Read the model definition and answer for the solid it produces. Units are mm, in the model's axes. A direction names the side the tool comes from. Give positions to 0.01 mm unless a question says otherwise; leave off trailing zeros. Loops run counter-clockwise (first coordinate to the right, second up) from the corner with the lowest first, then second, coordinate; pieces in that order, holes last. Notation, with made-up numbers: (81.5, 13.25) - (87.5, 13.25) arc R5 cw to (87.5, 20.25) - close; hole circle Ø8 at (6.25, -30). An arc over 180 degrees is marked (long way). Use a Markdown table: item, result. Add a question column.
Item 1: A cutting plane is placed at A-A (x = 0). Determine the outline of the cut face in (y, z), plus the area to 3 significant figures.
Item 2: Which of the six approach directions +Z, -Z, +X, -X, +Y, -Y give full straight-line access (tool end or side, diameter ignored) to faces 4 (the face through (19.48, 3.76, -21.04)), 5 (the face through (-26, 32, 12.7)), 6 (the face through (20.863, 59.743, -21.474))?
Item 3: Consider probe 1 along Z at (x, y) = (0, 49); probe 2 along Y at (x, z) = (-23, 12). Determine where each line is inside the solid, lowest interval first. Write a range as [from, to].
Item 4: A cutting plane is placed at C-C (y = 44.5). Determine the outline of the cut face in (x, z).
Item 5: Each of these flat-tipped pins is pushed along its axis until it touches: P1, Ø12, axis at x = -2.5, y = 45, coming from the +Z side; P2, Ø2, axis at x = -20.43, z = 20.43, coming from the +Y side; P3, Ø8, axis at x = -24.5, y = 29.5, coming from the -Z side; P4, Ø13.5, axis at x = 12.5, z = -18, coming from the -Y side. Where does it stop, or does it pass through?
Item 6: A cutting plane is placed at B-B (z = 0). Determine the outline of the cut face in (x, y), plus the area to 3 significant figures.
Item 7: A cutting plane is placed at D-D (z = 15.5). Determine the outline of the cut face in (x, y).
Item 8: For a pull along X with two mould halves and no side action, classify faces 1 (the face through (0, 25.4, -26)), 2 (the face through (-6.883, 31.306, 30.995)), 3 (the face through (20.37, 55.32, 20.24)) as +X half, -X half, draft (parallel to the pull), parting line (faces both ways), or undercut.
from build123d import *

# Parameters (mm, degrees)
SKETCH1_R                      = 31.75
SKETCH1_R_2                    = 25.4
BOSS_EXTRUDE1_DEPTH            = 63.5
F_4_40_TAPPED_HOLE1_AT_2_COUNT = 2
F_4_40_TAPPED_HOLE1_AT_2_PITCH = 40.860165351
F_4_40_TAPPED_HOLE1_AT_3_COUNT = 2
F_4_40_TAPPED_HOLE1_AT_3_PITCH = 57.785
F_4_40_TAPPED_HOLE1_AT_4_COUNT = 2
F_4_40_TAPPED_HOLE1_AT_4_PITCH = 40.860165351
SKETCH4_W                      = 112.670227293
SKETCH4_H                      = 56.447090519
CUT_EXTRUDE1_DEPTH             = 12.7


with BuildPart() as part:
    # Sketch1 → Boss-Extrude1 (new body)
    with BuildSketch(Plane(origin=(0, 0, 0), x_dir=(1, 0, 0), z_dir=(0, 1, 0))):
        Circle(SKETCH1_R)
        Circle(SKETCH1_R_2, mode=Mode.SUBTRACT)
    extrude(amount=BOSS_EXTRUDE1_DEPTH)

    # Sketch2 → #4-40 Tapped Hole1 (revolve, cut)
    with BuildSketch(Plane(origin=(-20.430082675, 0, 20.430082675), x_dir=(0, 0, -1), z_dir=(1, 0, 0))):
        Polygon((0, 0), (0, 8.299152758), (1.1303, 7.62), (1.1303, 0), align=None)
    f_4_40_tapped_hole1 = revolve(axis=Axis((-20.430082675, -6.35, 20.430082675), (0, 1, 0)), mode=Mode.SUBTRACT)

    # #4-40 Tapped Hole1 at 2: #4-40 Tapped Hole1 ×2
    with Locations(*[(i * F_4_40_TAPPED_HOLE1_AT_2_PITCH, 0, 0) for i in range(1, F_4_40_TAPPED_HOLE1_AT_2_COUNT)]):
        add(f_4_40_tapped_hole1, mode=Mode.SUBTRACT)

    # #4-40 Tapped Hole1 at 3: #4-40 Tapped Hole1 ×2
    with Locations(*[Vector(0.707106781, 0, -0.707106781) * (i * F_4_40_TAPPED_HOLE1_AT_3_PITCH) for i in range(1, F_4_40_TAPPED_HOLE1_AT_3_COUNT)]):
        add(f_4_40_tapped_hole1, mode=Mode.SUBTRACT)

    # #4-40 Tapped Hole1 at 4: #4-40 Tapped Hole1 ×2
    with Locations(*[(0, 0, -i * F_4_40_TAPPED_HOLE1_AT_4_PITCH) for i in range(1, F_4_40_TAPPED_HOLE1_AT_4_COUNT)]):
        add(f_4_40_tapped_hole1, mode=Mode.SUBTRACT)

    # Sketch4 → Cut-Extrude1 (cut)
    with BuildSketch(Plane(origin=(0, 25.4, 0), x_dir=(1, 0, 0), z_dir=(0, 1, 0))):
        with Locations((1.62115564, 15.52354526)):
            Rectangle(SKETCH4_W, SKETCH4_H)
    extrude(amount=CUT_EXTRUDE1_DEPTH, mode=Mode.SUBTRACT)

    # Mirror1: #4-40 Tapped Hole1 across plane
    add(f_4_40_tapped_hole1.mirror(Plane.ZX.offset(31.75)), mode=Mode.SUBTRACT)

    # Mirror1 copy 1 sketch → Mirror1 copy 1 (revolve, cut)
    with BuildSketch(Plane(origin=(20.430082675, 63.5, 20.430082675), x_dir=(0, 0, -1), z_dir=(1, 0, 0))):
        Polygon((0, 0), (0, -8.299152758), (1.1303, -7.62), (1.1303, 0), align=None)
    revolve(axis=Axis((20.430082675, 69.85, 20.430082675), (0, 1, 0)), mode=Mode.SUBTRACT)

    # Mirror1 copy 2 sketch → Mirror1 copy 2 (revolve, cut)
    with BuildSketch(Plane(origin=(20.430082675, 63.5, -20.430082675), x_dir=(0, 0, -1), z_dir=(1, 0, 0))):
        Polygon((0, 0), (0, -8.299152758), (1.1303, -7.62), (1.1303, 0), align=None)
    revolve(axis=Axis((20.430082675, 69.85, -20.430082675), (0, 1, 0)), mode=Mode.SUBTRACT)

    # Mirror1 copy 3 sketch → Mirror1 copy 3 (revolve, cut)
    with BuildSketch(Plane(origin=(-20.430082675, 63.5, -20.430082675), x_dir=(0, 0, -1), z_dir=(1, 0, 0))):
        Polygon((0, 0), (0, -8.299152758), (1.1303, -7.62), (1.1303, 0), align=None)
    revolve(axis=Axis((-20.430082675, 69.85, -20.430082675), (0, 1, 0)), mode=Mode.SUBTRACT)


solid = part.part
Geometry says:
| question | item | result |
|---|---|---|
| 1 | outline | (0, -31.75) - (25.4, -31.75) - (25.4, -25.4) - (0, -25.4) - close; (0, 25.4) - (63.5, 25.4) - (63.5, 31.75) - (0, 31.75) - close; (38.1, -31.75) - (63.5, -31.75) - (63.5, -25.4) - (38.1, -25.4) - close |
| 1 | area | 726 mm² |
| 2 | face 4 | -Y |
| 2 | face 5 | -Z, +X, -X |
| 2 | face 6 | +Y |
| 3 | probe 1 | [-31.75, -25.4], [25.4, 31.75] |
| 3 | probe 2 | [0, 25.4], [38.1, 63.5] |
| 4 | outline | circle Ø63.5 at (0, 0); hole circle Ø50.8 at (0, 0) |
| 5 | P1 | z = 31.75 |
| 5 | P2 | y = 55.8 |
| 5 | P3 | z = 12.7 |
| 5 | P4 | y = 0 |
| 6 | outline | (-31.75, 0) - (-25.4, 0) - (-25.4, 25.4) - (-31.75, 25.4) - close; (-31.75, 38.1) - (-25.4, 38.1) - (-25.4, 63.5) - (-31.75, 63.5) - close; (25.4, 0) - (31.75, 0) - (31.75, 25.4) - (25.4, 25.4) - close; (25.4, 38.1) - (31.75, 38.1) - (31.75, 63.5) - (25.4, 63.5) - close |
| 6 | area | 645 mm² |
| 7 | outline | (-27.71, 0) - (-20.12, 0) - (-20.12, 63.5) - (-27.71, 63.5) - close; (20.12, 0) - (27.71, 0) - (27.71, 63.5) - (20.12, 63.5) - close |
| 8 | face 1 | draft |
| 8 | face 2 | parting line |
| 8 | face 3 | undercut |
